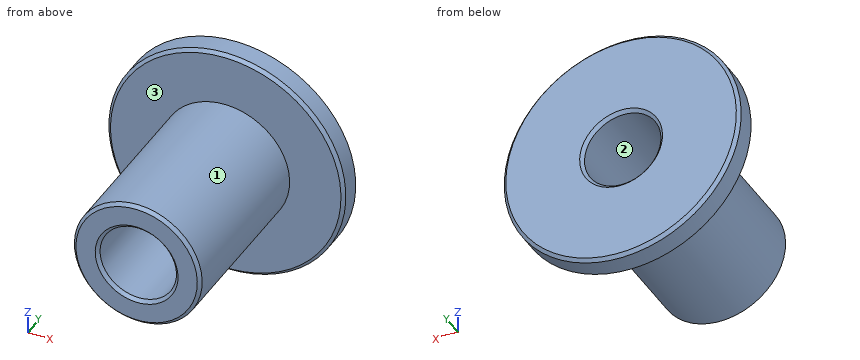
```python
from build123d import *

# Parameters (mm, degrees)
CHANFREIN1_SIZE = 0.25


with BuildPart() as part:
    # Esquisse1 → Base-Révolution (revolve)
    with BuildSketch(Plane.XY, mode=Mode.PRIVATE) as base_r_volution_sk:
        Polygon((2.975, 14.5), (2.975, 30), (9.225, 30), (9.225, 28), (4.975, 28), (4.975, 14.5), align=None)
    revolve(base_r_volution_sk.sketch.rotate(Axis((0, 30, 0), (0, -1, 0)), 90), axis=Axis((0, 30, 0), (0, -1, 0)))

    # Chanfrein1
    chanfrein1_edges = [part.edges().sort_by_distance(p)[0] for p in [
        (0, 14.5, -2.975),
        (0, 30, -2.975),
        (0, 30, -9.225),
        (0, 28, -9.225),
        (0, 14.5, -4.975),
    ]]
    chamfer(chanfrein1_edges, length=CHANFREIN1_SIZE)


solid = part.part
```
The listing builds one solid part. Answer for the finished solid, in the listing's coordinates (mm). Face numbers are marked on the shaded views. Round coordinates to 2 decimals unless told otherwise and drop trailing zeros. Loops run counter-clockwise (first coordinate to the right, second up) from the corner with the lowest first, then second, coordinate; pieces in that order, holes last. Notation, with made-up numbers: (27.25, -35.5) - (42.25, -35.5) arc R26 ccw to (42.25, -14.5) - close; hole circle Ø9 at (41.25, -25). An arc over 180 degrees is marked (long way). Return JSON: item names as keys, results as strings. Group by question number.
1. Consider probe 1 along X at (y, z) = (20, 0) (3 decimals); probe 2 along Y at (x, z) = (-0.25, 5.25); probe 3 along X at (y, z) = (29, -2). Determine where each line is inside the solid, lowest interval first.
2. Each of these flat-tipped pins is pushed along its axis until it touches: P1, Ø8, axis at y = 21.5, z = 0, coming from the +X side (3 decimals); P2, Ø2, axis at x = 5, y = 16, coming from the +Z side; P3, Ø4, axis at y = 23, z = -5, coming from the +X side. Where does it stop, or does it pass through?
3. The part is cut by section B-B on x = 0. Determine the outline of the cut face in (y, z) (3 decimals).
4. The part is cut by section A-A on z = 0. Determine the outline of the cut face in (x, y) (3 decimals).
5. The part is cut by section C-C on y = 23.25. Determine the outline of the cut face in (x, z) (3 decimals), then the cut area to 3 significant figures.
6. The mould has two halves that part along X. Classify the marked faces 1, 2 and 3: pulls with the +X half, pulls with the -X half, needs draft (parallel to the pull), parting line crosses it, or undercut.
Resolved:
{
 "1": {"probe 1": "x = -4.975 to -2.975, 2.975 to 4.975", "probe 2": "y = 28 to 30", "probe 3": "x = -9.01 to -2.2, 2.2 to 9.01"},
 "2": {"P1": "stops at x = 4.975", "P2": "stops at z = 2.96", "P3": "stops at x = 3.97"},
 "3": {"outline": "(14.5, -4.725) - (14.75, -4.975) - (28, -4.975) - (28, -8.975) - (28.25, -9.225) - (29.75, -9.225) - (30, -8.975) - (30, -3.225) - (29.75, -2.975) - (14.75, -2.975) - (14.5, -3.225) - close; (14.5, 3.225) - (14.75, 2.975) - (29.75, 2.975) - (30, 3.225) - (30, 8.975) - (29.75, 9.225) - (28.25, 9.225) - (28, 8.975) - (28, 4.975) - (14.75, 4.975) - (14.5, 4.725) - close"},
 "4": {"outline": "(-9.225, 28.25) - (-8.975, 28) - (-4.975, 28) - (-4.975, 14.75) - (-4.725, 14.5) - (-3.225, 14.5) - (-2.975, 14.75) - (-2.975, 29.75) - (-3.225, 30) - (-8.975, 30) - (-9.225, 29.75) - close; (2.975, 14.75) - (3.225, 14.5) - (4.725, 14.5) - (4.975, 14.75) - (4.975, 28) - (8.975, 28) - (9.225, 28.25) - (9.225, 29.75) - (8.975, 30) - (3.225, 30) - (2.975, 29.75) - close"},
 "5": {"outline": "circle Ø9.95 at (0, 0); hole circle Ø5.95 at (0, 0)", "area": "50.0 mm²"},
 "6": {"face 1": "parting line crosses it", "face 2": "undercut", "face 3": "needs draft"}
}
